Part model, mm, in its own coordinate system. Face numbers are marked on the shaded views. A direction names the side the tool comes from. Coordinates: 2 decimals unless noted, no trailing zeros. Order: outer loops, then holes, each group sorted by start corner. A loop starts at its lowest first (then second) coordinate and runs counter-clockwise, first axis right, second up. Notation, with made-up numbers: M 79,-28 L 133,-28 A28 cw 133,7 Z; hole C 56.25,47 d10. An arc over 180 degrees is marked long. Answer in a Markdown table with one row per item. Add a question column.
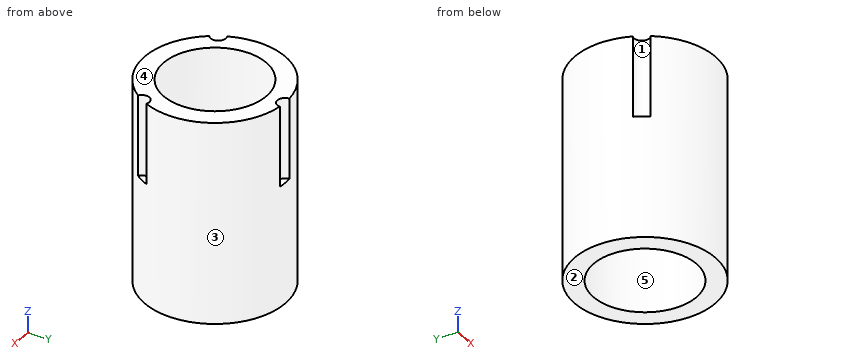
from build123d import *

# Parameters (mm, degrees)
ESQUISSE1_R             = 17.5
BOSS_EXTRU_1_DEPTH      = 50
ESQUISSE4_R             = 12.8
ENL_V_MAT_EXTRU_1_DEPTH = 50
ESQUISSE5_R             = 1.9
ENL_V_MAT_EXTRU_2_DEPTH = 20


with BuildPart() as part:
    # Esquisse1 → Boss.-Extru.1 (new body)
    with BuildSketch(Plane.XY):
        Circle(ESQUISSE1_R)
    extrude(amount=BOSS_EXTRU_1_DEPTH)

    # Esquisse4 → Enlèv. mat.-Extru.1 (cut)
    with BuildSketch(Plane.XY.offset(50)):
        Circle(ESQUISSE4_R)
    extrude(amount=-ENL_V_MAT_EXTRU_1_DEPTH, mode=Mode.SUBTRACT)

    # Esquisse5 → Enlèv. mat.-Extru.2 (cut)
    with BuildSketch(Plane.XY.offset(50)):
        with Locations((0, 17.5)):
            Circle(ESQUISSE5_R)
        with Locations((15.155444566, -8.75)):
            Circle(ESQUISSE5_R)
        with Locations((-15.155444566, -8.75)):
            Circle(ESQUISSE5_R)
    extrude(amount=-ENL_V_MAT_EXTRU_2_DEPTH, mode=Mode.SUBTRACT)


solid = part.part
(1) Slice it at D-D (x = 7). List the corners of the cut face in (y, z), and give its area (3 significant figures).
(2) Drop flat-ended pins along their axis: P1, Ø1, axis at y = -2, z = 27.5, coming from the +X side; P2, Ø0.6, axis at x = 0, y = 17, coming from the +Z side; P3, Ø4, axis at y = 11.5, z = 9.5, coming from the +X side. Give the stop position or say it passes through.
(3) Slice it at A-A (y = 0). List the corners of the cut face in (x, z).
(4) Slice it at B-B (x = 0). List the corners of the cut face in (y, z).
(5) 3-axis set-ups, long thin cutter, end or side, ignore diameter. For the marked faces 1 and 2: which of +Z, -Z, +X, -X, +Y, -Y reach the whole face in a straight line?
(6) Wall check: line 1 (Y direction, x = 0, z = 17); line 2 (Y direction, x = -11, z = 36); line 3 (X direction, y = 1.5, z = 3). Give the ranges that are in metal, low to high.
(7) Pull direction Y, two halves, no side cores. Call the marked faces 3, 4 and 5: pulls with the +Y half, pulls with the -Y half, needs draft (parallel to the pull), parting line crosses it, or undercut.
(8) Slice it at C-C (z = 12). List the corners of the cut face in (x, y).
Computed:
| question | item | result |
|---|---|---|
| 1 | outline | M -16.04,0 L -10.72,0 L -10.72,50 L -16.04,50 Z; M 10.72,0 L 16.04,0 L 16.04,50 L 10.72,50 Z |
| 1 | area | 532 mm^2 |
| 2 | P1 | stops at x = 17.44 |
| 2 | P2 | stops at z = 30 |
| 2 | P3 | stops at x = 14.7 |
| 3 | outline | M -17.5,0 L -12.8,0 L -12.8,50 L -17.5,50 Z; M 12.8,0 L 17.5,0 L 17.5,50 L 12.8,50 Z |
| 4 | outline | M -17.5,0 L -12.8,0 L -12.8,50 L -17.5,50 Z; M 12.8,0 L 17.5,0 L 17.5,30 L 15.6,30 L 15.6,50 L 12.8,50 Z |
| 5 | face 1 | +Z |
| 5 | face 2 | -Z, +X, -X, +Y, -Y |
| 6 | line 1 | y = -17.5 to -12.8, 12.8 to 17.5 |
| 6 | line 2 | y = -13.61 to -6.55, 6.55 to 13.61 |
| 6 | line 3 | x = -17.44 to -12.71, 12.71 to 17.44 |
| 7 | face 3 | parting line crosses it |
| 7 | face 4 | needs draft |
| 7 | face 5 | undercut |
| 8 | outline | C 0,0 d35; hole C 0,0 d25.6 |
